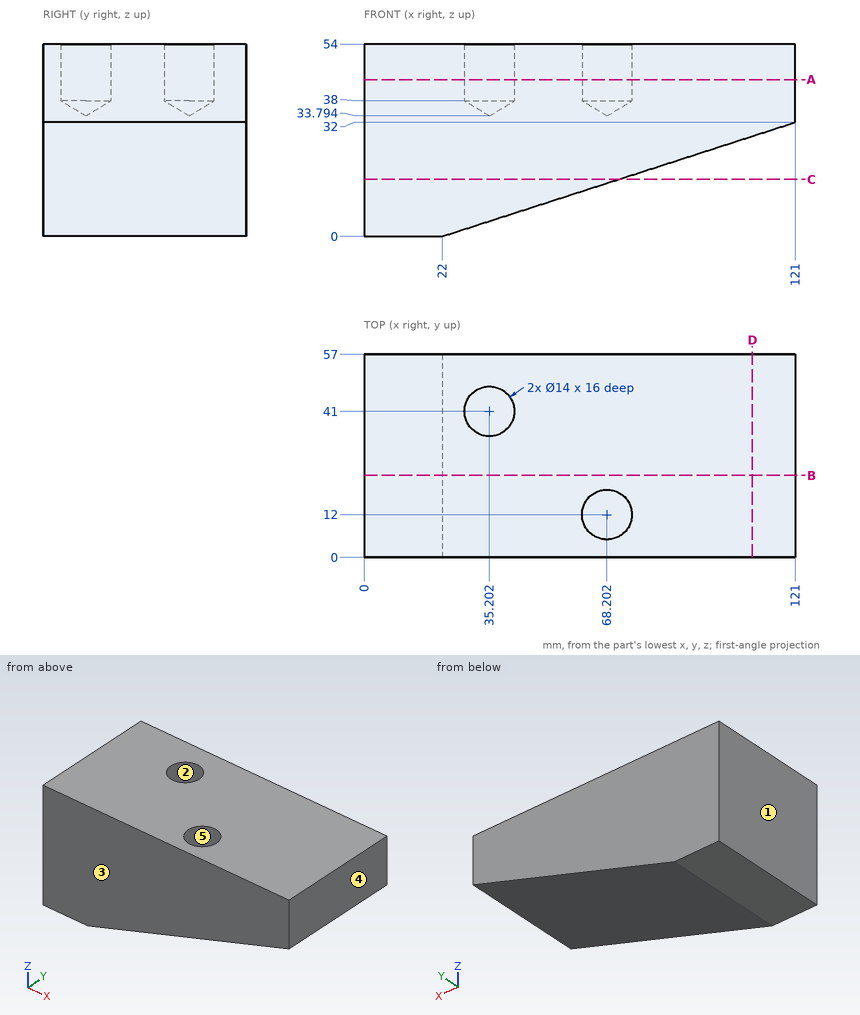
Design review of the part shown in the three views and the two pictorial views. Dimensions are in mm from the part's minimum x, y and z. A direction names the side the tool comes from. Coordinates: 2 decimals unless noted, no trailing zeros. Write each loop counter-clockwise with the first axis right and the second up, starting at its lowest first coordinate (ties: lowest second). Pieces come first, ordered by that corner, then holes.
1) We need section D-D on x = 109. State the section outline as (y, z) points, then the cut area to 4 significant figures.
2) To check wall thickness, follow probe 1 along Y at (x, z) = (35, 46.5); probe 2 along X at (y, z) = (12, 50); probe 3 along X at (y, z) = (41, 46.5). State the ranges of each line that lie inside material, in increasing order.
3) Clearance check with flat-ended pins moving along their axes: pin 1 Ø12.5 at (x, y) = (35.2, 41) entering from -Z; pin 2 Ø5 at (x, y) = (56.5, 47) entering from -Z; pin 3 Ø11 at (x, y) = (68.2, 12) entering from +Z. State where each tip first meets the part, or that it passes through.
4) We need section B-B on y = 23. State the section outline as (x, z) points, then the cut area to 3 significant figures.
5) Machinability: for the marked faces 1 and 2, which of the approach directions +Z, -Z, +X, -X, +Y, -Y give a long, thin tool a straight path to every point of the face, cutting with its end or side? Answer none if there is none.
6) We need section C-C on z = 16. State the section outline as (x, y) points, then the cut area to 3 significant figures.
7) The part is to be moulded in two halves that separate along X. For the marked faces 3, 4 and 5, say which applies: pulls with the +X half, pulls with the -X half, needs draft (parallel to the pull), parting line crosses it, or undercut.
8) We need section A-A on z = 44. State the section outline as (x, y) points, then the cut area to 3 significant figures.
Answer list:
1. outline: (0, 28.12) - (57, 28.12) - (57, 54) - (0, 54) - close
1. area: 1,475 mm2
2. probe 1: y = 0 to 34, 48 to 57
2. probe 2: x = 0 to 61.2, 75.2 to 121
2. probe 3: x = 0 to 28.2, 42.2 to 121
3. pin 1: stops at z = 2.25
3. pin 2: stops at z = 10.34
3. pin 3: stops at z = 37.1
4. outline: (0, 0) - (22, 0) - (121, 32) - (121, 54) - (0, 54) - close
4. area: 4,950 mm2
5. face 1: +Z, -Z, -X, +Y, -Y
5. face 2: +Z
6. outline: (0, 0) - (71.5, 0) - (71.5, 57) - (0, 57) - close
6. area: 4,080 mm2
7. face 3: needs draft
7. face 4: pulls with the +X half
7. face 5: undercut
8. outline: (0, 0) - (121, 0) - (121, 57) - (0, 57) - close; hole circle Ø14 at (35.2, 41); hole circle Ø14 at (68.2, 12)
8. area: 6,590 mm2
